For this review, take the finished solid that the model builds, in its own axes (mm). Coordinates: 2 decimals unless noted, no trailing zeros. Write each loop counter-clockwise with the first axis right and the second up, starting at its lowest first coordinate (ties: lowest second). Pieces come first, ordered by that corner, then holes.
1) Insertion check: P1, Ø6, axis at x = 13.5, z = -8.5, coming from the +Y side; P2, Ø1.5, axis at x = 13.5, y = 3, coming from the +Z side; P3, Ø2, axis at x = 4.5, y = 3, coming from the -Z side; P4, Ø3, axis at x = -13.5, y = 3, coming from the -Z side. Each pin has a flat end and moves straight along its axis. Give the tip position at first contact, or say it passes through.
2) We need section D-D on z = -8. Write out the cut boundary in (x, y).
3) To check wall thickness, follow line 1 along X through (y, z) = (4.5, 7); line 2 along X through (y, z) = (3, 46); line 3 along Y through (x, z) = (-13.5, 46.75). State the ranges of each line that lie inside material, in increasing order.
4) We need section B-B on z = 45.5. Write out the cut boundary in (x, y), then the cut area to 3 significant figures.
5) We need section A-A on z = 2. Write out the cut boundary in (x, y).
6) We need section C-C on y = 5. Write out the cut boundary in (x, z).
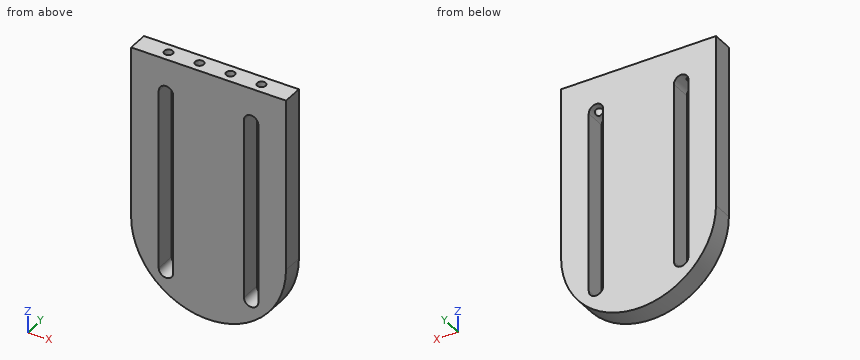
from build123d import *

# Parameters (mm, degrees)
EXTRUDE_1_DEPTH     = 6
CUT_EXTRUDE_1_DEPTH = 56.156595254
M3X0_51_D           = 2.5
M3X0_51_DEPTH       = 8.5
M3X0_51_TIP         = 0.751075774


with BuildPart() as part:
    # Эскиз1 → Бобышка-Вытянуть1 (new body)
    with BuildSketch(Plane(origin=(0, 0, 0), x_dir=(1, 0, 0), z_dir=(0, 1, 0))):
        with BuildLine():
            Line((-22.5, 0), (-22.5, -50))
            Line((-22.5, -50), (22.5, -50))
            Line((22.5, -50), (22.5, 0))
            ThreePointArc((22.5, 0), (0, 22.5), (-22.5, 0))
        make_face()
    extrude(amount=EXTRUDE_1_DEPTH)

    # Эскиз2 → Вырез-Вытянуть1 (cut, through all)
    with BuildSketch(Plane(origin=(0, 6, 0), x_dir=(1, 0, 0), z_dir=(0, 1, 0))):
        with BuildLine():
            Line((-10.274368671, 12.374368671), (-10.274368671, -40))
            ThreePointArc((-10.274368671, -40), (-12.374368671, -42.1), (-14.474368671, -40))
            Line((-14.474368671, -40), (-14.474368671, 12.374368671))
            ThreePointArc((-14.474368671, 12.374368671), (-12.374368671, 14.474368671), (-10.274368671, 12.374368671))
        make_face()
        with BuildLine():
            Line((10.274368671, 12.374368671), (10.274368671, -40))
            ThreePointArc((10.274368671, -40), (12.374368671, -42.1), (14.474368671, -40))
            Line((14.474368671, -40), (14.474368671, 12.374368671))
            ThreePointArc((14.474368671, 12.374368671), (12.374368671, 14.474368671), (10.274368671, 12.374368671))
        make_face()
    extrude(amount=-CUT_EXTRUDE_1_DEPTH, mode=Mode.SUBTRACT)

    # Отверстие обработанное метчиком M3x0.51
    with Locations(Plane.XY.offset(50)):
        with Locations((-13.5, 3), (-4.5, 3), (4.5, 3), (13.5, 3)):
            Hole(M3X0_51_D / 2, depth=M3X0_51_DEPTH)
            with Locations((0, 0, -(M3X0_51_DEPTH + M3X0_51_TIP / 2))):  # 118° drill point
                Cone(0, M3X0_51_D / 2, M3X0_51_TIP, mode=Mode.SUBTRACT)


solid = part.part
Result:
1. P1: stops at y = 6
1. P2: stops at z = 41.2
1. P3: stops at z = -22.23
1. P4: stops at z = -19.03
2. outline: (-21.03, 0) - (-14.47, 0) - (-14.47, 6) - (-21.03, 6) - close; (-10.27, 0) - (10.27, 0) - (10.27, 6) - (-10.27, 6) - close; (14.47, 0) - (21.03, 0) - (21.03, 6) - (14.47, 6) - close
3. line 1: x = -22.5 to -14.47, -10.27 to 10.27, 14.47 to 22.5
3. line 2: x = -22.5 to -14.75, -12.25 to -5.75, -3.25 to 3.25, 5.75 to 12.25, 14.75 to 22.5
3. line 3: y = 0 to 1.75, 4.25 to 6
4. outline: (-22.5, 0) - (22.5, 0) - (22.5, 6) - (-22.5, 6) - close; hole circle Ø2.5 at (-13.5, 3); hole circle Ø2.5 at (-4.5, 3); hole circle Ø2.5 at (4.5, 3); hole circle Ø2.5 at (13.5, 3)
4. area: 250 mm2
5. outline: (-22.5, 0) - (-14.47, 0) - (-14.47, 6) - (-22.5, 6) - close; (-10.27, 0) - (10.27, 0) - (10.27, 6) - (-10.27, 6) - close; (14.47, 0) - (22.5, 0) - (22.5, 6) - (14.47, 6) - close
6. outline: (-22.5, 0) arc R22.5 ccw to (22.5, 0) - (22.5, 50) - (-22.5, 50) - close; hole (-14.47, -12.37) arc R2.1 ccw to (-10.27, -12.37) - (-10.27, 40) arc R2.1 ccw to (-14.47, 40) - close; hole (10.27, -12.37) arc R2.1 ccw to (14.47, -12.37) - (14.47, 40) arc R2.1 ccw to (10.27, 40) - close
